from build123d import *

# Parameters (mm, degrees)
F2_T = -50.8


# Not quite as in the source:
# - a fillet or chamfer that OpenCascade refuses, or shapes differently, is made with other operations: its cross-section is extruded or revolved along the edge and cut away or added


with BuildPart() as f1:
    # F0 (on Front) → F1 (revolve)
    with BuildSketch(Plane.XZ):
        with BuildLine():
            Line((-762, 0), (0, 0))
            Line((0, 0), (0, 1778))
            Line((0, 1778), (-635, 1778))
            ThreePointArc((-635, 1778), (-537.4071698995, 877.4933692785), (-762, 0))
        make_face()
    revolve(axis=Axis((0, 0, 889), (0, 0, -1)))

    # F2
    f2_openings = [f1.faces().sort_by_distance(p)[0] for p in [
        (0, 0, 1778),
    ]]
    offset(amount=F2_T, openings=f2_openings)

    # F3: fillet of radius 25.4 on 2 edges, made by hand

    # F3_s1 → F3_t2 (revolve, cut)
    with BuildSketch(Plane.XZ):
        with BuildLine():
            ThreePointArc((-601.2462046198, 1778), (-585.9068056848, 1772.845069531), (-576.7936693441, 1759.4726645916))
            ThreePointArc((-576.7936693441, 1759.4726645916), (-579.4173103836, 1768.7412417508), (-582.075394382, 1778))
            Line((-582.075394382, 1778), (-601.2462046198, 1778))
        make_face()
    revolve(axis=Axis((0, 0, 1778), (0, 0, 1)), mode=Mode.SUBTRACT)

    # F3_s3 → F3_t4 (revolve, cut)
    with BuildSketch(Plane.XZ):
        with BuildLine():
            ThreePointArc((-625.6987398956, 1745.7273354084), (-621.4912741508, 1767.939398935), (-601.2462046198, 1778))
            Line((-601.2462046198, 1778), (-635, 1778))
            ThreePointArc((-635, 1778), (-630.296026904, 1761.8790416292), (-625.6987398956, 1745.7273354084))
        make_face()
    revolve(axis=Axis((0, 0, 1778), (0, 0, -1)), mode=Mode.SUBTRACT)


solid = f1.part
Geometry check sheet. Reference: the model listing, model coordinates, mm. Give positions to 0.01 mm unless a question says otherwise; leave off trailing zeros. Order: outer loops, then holes, each group sorted by start corner. A loop starts at its lowest first (then second) coordinate and runs counter-clockwise, first axis right, second up. Notation, with made-up numbers: M 43,4.5 L 97,4.5 A22 cw 97,41.5 Z; hole C 15,37.5 d6. An arc over 180 degrees is marked long. Use a Markdown table: item, result.
Item 1: Material ranges on line 1 along X through (y, z) = (157.5, 126.5); line 2 along Y through (x, z) = (315, 202); line 3 along Z through (x, y) = (-197, 159), recorded low to high.
Answers follow:
| item | result |
|---|---|
| line 1 | x = -690.37 to -634.32, 634.32 to 690.37 |
| line 2 | y = -602.3 to -540.75, 540.75 to 602.3 |
| line 3 | z = 0 to 50.8 |
Item 2: Section check A-A (z = 927.5). Record the cut outline in (x, y).
Answers follow:
| item | result |
|---|---|
| outline | C 0,0 d1068.66; hole C 0,0 d966.93 |
Item 3: Draft check along Z on faces 1 (the flat face through (10, 10, 50.8)), 2 (the flat face through (11, 11, 0)). Enter one of: +Z half, -Z half, draft (parallel to the pull), parting line (faces both ways), or undercut.
Answers follow:
| item | result |
|---|---|
| face 1 | undercut |
| face 2 | -Z half |
Item 4: Section check C-C (z = 1220.5). Record the cut outline in (x, y).
Answers follow:
| item | result |
|---|---|
| outline | C 0,0 d1072.25; hole C 0,0 d970.45 |
Item 5: Section check B-B (y = 567). State how many separate pieces and enclosed holes the cut face has, and give its area (3 significant figures).
Answers follow:
| item | result |
|---|---|
| separate pieces | 2 |
| enclosed holes | 1 |
| area | 303,000 mm2 |
Item 6: Depth check by flat-ended pin: P1, Ø2, axis at x = -64, y = -577.5, coming from the +Z side; P2, Ø5, axis at x = 380, z = 332, coming from the +Y side; P3, Ø8, axis at x = 50, y = 118.5, coming from the -Z side; P4, Ø1.5, axis at x = -130.5, z = 732, coming from the +Y side. Enter the tip coordinate at first touch or a pass-through.
Answers follow:
| item | result |
|---|---|
| P1 | stops at z = 1769.22 |
| P2 | stops at y = 513.38 |
| P3 | stops at z = 0 |
| P4 | stops at y = 536.58 |
